Design review of the part built by this model. Coordinates are the model's own, in mm. Coordinates: 2 decimals unless noted, no trailing zeros. Loops run counter-clockwise (first coordinate to the right, second up) from the corner with the lowest first, then second, coordinate; pieces in that order, holes last. Notation, with made-up numbers: (-15, 36.5) -> (-9, 36.5) arc R26 cw to (-9, 53.5) -> close; hole circle Ø4 at (59.5, -32.75). An arc over 180 degrees is marked (long way). Use one line per item in the form item = value. Start each with the question number.
1. Consider section A-A (y = 0). State the section outline as (x, z) points.
2. The part is to be moulded in two halves that separate along X. For faces 1 (the face through (68.034, -36.032, 1.014)), 2 (the face through (24, 10, 2)), say which applies: released by +X, released by -X, zero draft, split by the parting line, or undercut.
3. Wall thickness on line 1 (Y direction, x = 25.5, z = 1.6); line 2 (X direction, y = 55, z = 1.55); line 3 (Y direction, x = 49, z = 0.1): over which ranges is each line inside the solid? List them lowest first. Write a range as from..to.
4. Consider section B-B (z = 0.95). State how many separate pieces and enclosed holes the cut face has, then the cut area to 3 significant figures.
5. For pin 1 (5 mm diameter, centred on x = 62.5, y = 9.5, fed in from -Z), flat-tipped, find the tip position at first contact; note if it passes through.
from build123d import *

# Parameters (mm, degrees)
F0_W     = 100
F0_H     = 100
F0_R     = 2
F0_W_2   = 13
F0_H_2   = 22
F0_W_3   = 16.1784952506
F0_H_3   = 7.3538627476
F1_DEPTH = 2
F2_D     = 4
F2_DEPTH = 15
F2_TIP   = 1.2017212381


with BuildPart() as f1:
    # F0 (on Top) → F1 (new body)
    with BuildSketch(Plane.XY):
        with Locations((24.3766545396, 9.4889727443)):
            Rectangle(F0_W, F0_H)
        with Locations((25.2671993673, -33.7579216361)):
            Circle(F0_R, mode=Mode.SUBTRACT)
        with Locations((25.2671993673, -16.8789608181)):
            Rectangle(F0_W_2, F0_H_2, mode=Mode.SUBTRACT)
        with Locations((25.2671993673, 0)):
            Circle(F0_R, mode=Mode.SUBTRACT)
        with Locations((45.1880805272, 40.0074942991)):
            Rectangle(F0_W_3, F0_H_3, mode=Mode.SUBTRACT)
    extrude(amount=F1_DEPTH)

    # F2
    with Locations(Plane(origin=(0, 0, 0), x_dir=(1, 0, 0), z_dir=(0, 0, -1))):
        with Locations((-22.1756645401, -54.9460881411), (69.9414474967, 35.4310135335), (69.9414474967, -54.9460881411), (-22.1756645401, 35.4310135335)):
            Hole(F2_D / 2, depth=F2_DEPTH)
            with Locations((0, 0, -(F2_DEPTH + F2_TIP / 2))):  # 118° drill point
                Cone(0, F2_D / 2, F2_TIP, mode=Mode.SUBTRACT)


solid = f1.part
Geometry check:
q1.outline = (-25.62, 0) -> (23.27, 0) -> (23.27, 2) -> (-25.62, 2) -> close; (27.27, 0) -> (74.38, 0) -> (74.38, 2) -> (27.27, 2) -> close
q2.face_1 = undercut
q2.face_2 = zero draft
q3.line_1 = -40.51..-35.74, -31.77..-27.88, -5.88..-1.99, 1.99..59.49
q3.line_2 = -25.62..-24.17, -20.18..67.94, 71.94..74.38
q3.line_3 = -40.51..36.33, 43.68..59.49
q4.separate_pieces = 1
q4.enclosed_holes = 8
q4.area = 9,520 mm²
q5.pin_1 = 0
